Read the model definition and answer for the solid it produces. Units are mm, in the model's axes. A direction names the side the tool comes from. Give positions to 0.01 mm unless a question says otherwise; leave off trailing zeros. Loops run counter-clockwise (first coordinate to the right, second up) from the corner with the lowest first, then second, coordinate; pieces in that order, holes last. Notation, with made-up numbers: (24.25, -29) - (59.25, -29) arc R31 cw to (59.25, 6) - close; hole circle Ø5 at (-16.5, -37). An arc over 180 degrees is marked (long way). Write item = value, one per line. Start each with the question number.
from build123d import *

# Parameters (mm, degrees)
F0_W     = 50.8
F0_H     = 50.8
F1_DEPTH = 50.8
F2_W     = 36.0644307539
F2_H     = 25.4
F3_DEPTH = 25.4


with BuildPart() as f1:
    # F0 (on Right) → F1 (new body)
    with BuildSketch(Plane.YZ):
        with Locations((-1.3928227127, 5.918835211)):
            Rectangle(F0_W, F0_H)
    extrude(amount=F1_DEPTH)

    # F2 (on face) → F3 (cut)
    with BuildSketch(Plane.XY.offset(31.318835211)):
        with Locations((32.7677846231, -14.0928227127)):
            Rectangle(F2_W, F2_H)
    extrude(amount=-F3_DEPTH, mode=Mode.SUBTRACT)


solid = f1.part
1. A cutting plane is placed at B-B on y = -21. Give the vertices of the cut face in (x, z), and give its area (3 significant figures).
2. Given P1, Ø4, axis at y = 4.5, z = 13.5, coming from the -X side; P2, Ø12.5, axis at y = -19.5, z = 20.5, coming from the +X side, each flat-ended and moving along its own axis, determine where each tip first touches the part or whether it passes through.
3. A tool of negligible diameter and unlimited length cuts with its end or side. For faces 1 (the flat face through (33, -1.393, 19)), 2 (the flat face through (50.8, 4, 1)), from which of +Z, -Z, +X, -X, +Y, -Y can it reach the whole face along a straight path? Write none if from no direction.
4. A cutting plane is placed at A-A on z = 15.5. Give the vertices of the cut face in (x, y).
5. Consider line 1 along Z through (x, y) = (47.5, -9); line 2 along Y through (x, z) = (28.5, 15); line 3 along X through (y, z) = (-21, 16). Determine where each line is inside the solid, lowest interval first. Write a range as [from, to].
Reply:
q1.outline = (0, -19.48) - (50.8, -19.48) - (50.8, 5.92) - (14.74, 5.92) - (14.74, 31.32) - (0, 31.32) - close
q1.area = 1,660 mm^2
q2.P1 = 0
q2.P2 = 14.74
q3.face_1 = +Z, +X, -Y
q3.face_2 = +Z, -Z, +X, +Y, -Y
q4.outline = (0, -26.79) - (14.74, -26.79) - (14.74, -1.39) - (50.8, -1.39) - (50.8, 24.01) - (0, 24.01) - close
q5.line_1 = [-19.48, 5.92]
q5.line_2 = [-1.39, 24.01]
q5.line_3 = [0, 14.74]
